Read the model definition and answer for the solid it produces. Units are mm, in the model's axes. Coordinates: 2 decimals unless noted, no trailing zeros. Write each loop counter-clockwise with the first axis right and the second up, starting at its lowest first coordinate (ties: lowest second). Pieces come first, ordered by that corner, then holes.
(1) Section A-A on x = 0 is taken. Write down the section's boundary in (y, z).
(2) Section D-D on x = -3.5 is taken. Write down the section's boundary in (y, z).
(3) Section C-C on y = -0.3 is taken. Write down the section's boundary in (x, z), then the cut area to 3 significant figures.
(4) Given pin 1 (9 mm diameter, centred on x = 0, z = -19, fed in from +Y), flat-ended and moving along its own axis, determine where the tip first touches the part or whether it passes through.
(5) Find the intervals of material crossed by probe 1 along Z at (x, y) = (0, 0.45); probe 2 along X at (y, z) = (-0.2, 19); probe 3 along Z at (x, y) = (-3.5, 0.7), in increasing order.
(6) Section B-B on z = -21 is taken. Write down the section's boundary in (x, y).
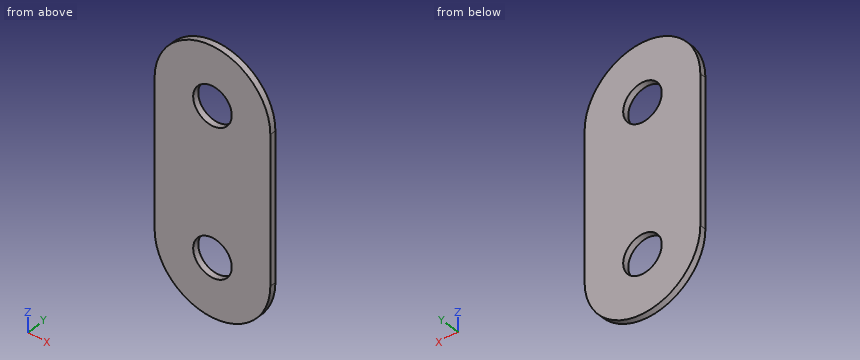
from build123d import *

# Parameters (mm, degrees)
BOSS_EXTRUDE2_DEPTH     = 0.8
CUT_EXTRUDE2_DEPTH      = 38.170418346
CUT_EXTRUDE2_DEPTH_BACK = 38.170418346
SKETCH7_R               = 5


with BuildPart() as part:
    # Sketch6 → Boss-Extrude2 (new, symmetric)
    with BuildSketch(Plane(origin=(0, 0, 0), x_dir=(1, 0, 0), z_dir=(0, 1, 0))):
        with BuildLine():
            Line((-15, 19), (-15, -19))
            ThreePointArc((-15, -19), (0, -34), (15, -19))
            Line((15, -19), (15, 19))
            ThreePointArc((15, 19), (0, 34), (-15, 19))
        make_face()
    extrude(amount=BOSS_EXTRUDE2_DEPTH, both=True)

    # Sketch7 → Cut-Extrude2 (cut, two sides: drawn at the far end of the back side and taken through both)
    with BuildSketch(Plane(origin=(0, 0, 0), x_dir=(1, 0, 0), z_dir=(0, 1, 0)).offset(-CUT_EXTRUDE2_DEPTH_BACK)):
        with Locations(Location((0, 19, 0), (0, 0, 270))):
            Circle(SKETCH7_R)
        with Locations(Location((0, -19, 0), (0, 0, 270))):
            Circle(SKETCH7_R)
    extrude(amount=CUT_EXTRUDE2_DEPTH + CUT_EXTRUDE2_DEPTH_BACK, mode=Mode.SUBTRACT)


solid = part.part
Response:
1. outline: (-0.8, -34) - (0.8, -34) - (0.8, -24) - (-0.8, -24) - close; (-0.8, -14) - (0.8, -14) - (0.8, 14) - (-0.8, 14) - close; (-0.8, 24) - (0.8, 24) - (0.8, 34) - (-0.8, 34) - close
2. outline: (-0.8, -33.59) - (0.8, -33.59) - (0.8, -22.57) - (-0.8, -22.57) - close; (-0.8, -15.43) - (0.8, -15.43) - (0.8, 15.43) - (-0.8, 15.43) - close; (-0.8, 22.57) - (0.8, 22.57) - (0.8, 33.59) - (-0.8, 33.59) - close
3. outline: (-15, -19) arc R15 ccw to (15, -19) - (15, 19) arc R15 ccw to (-15, 19) - close; hole circle Ø10 at (0, -19); hole circle Ø10 at (0, 19)
3. area: 1,690 mm2
4. pin 1: passes through
5. probe 1: z = -34 to -24, -14 to 14, 24 to 34
5. probe 2: x = -15 to -5, 5 to 15
5. probe 3: z = -33.59 to -22.57, -15.43 to 15.43, 22.57 to 33.59
6. outline: (-14.87, -0.8) - (-4.58, -0.8) - (-4.58, 0.8) - (-14.87, 0.8) - close; (4.58, -0.8) - (14.87, -0.8) - (14.87, 0.8) - (4.58, 0.8) - close
